from build123d import *

# Parameters (mm, degrees)
F0_R     = 3
F1_DEPTH = 6.4
F4_DEPTH = 3.2
F5_SIZE  = 2


with BuildPart() as f1:
    # F0 (on Top) → F1 (new body)
    with BuildSketch(Plane.XY):
        with BuildLine():
            Line((-69.9830439783, 22.2635182233), (-43.4754125815, 17.5895076134))
            Line((-43.4754125815, 17.5895076134), (-75.4919030254, 33.0095051449))
            ThreePointArc((-75.4919030254, 33.0095051449), (-71.3637669974, 29.3201416884), (-69.8311215084, 24))
            ThreePointArc((-69.8311215084, 24), (-69.8691745275, 23.1284425725), (-69.9830439783, 22.2635182233))
        make_face()
        with BuildLine():
            Line((-90, -10), (-30, -10))
            ThreePointArc((-30, -10), (-37.0710678119, -7.0710678119), (-40, 0))
            Line((-40, 0), (-57, 0))
            ThreePointArc((-57, 0), (-60, -3), (-63, 0))
            Line((-63, 0), (-80, 0))
            ThreePointArc((-80, 0), (-82.9289321881, -7.0710678119), (-90, -10))
        make_face()
        with BuildLine():
            Line((-78.0946397318, 33.8480775301), (-107.6388723221, 39.0575228601))
            ThreePointArc((-107.6388723221, 39.0575228601), (-101.7149096676, 35.6373214269), (-99.3753540988, 29.20944533))
            ThreePointArc((-99.3753540988, 29.20944533), (-99.4134071179, 28.3378879025), (-99.5272765687, 27.4729635533))
            Line((-99.5272765687, 27.4729635533), (-89.6791990386, 25.7364817767))
            ThreePointArc((-89.6791990386, 25.7364817767), (-85.566885872, 32.1915204429), (-78.0946397318, 33.8480775301))
        make_face()
        with BuildLine():
            ThreePointArc((-89.6791990386, 25.7364817767), (-81.5676032851, 14.1519224699), (-69.9830439783, 22.2635182233))
            Line((-69.9830439783, 22.2635182233), (-76.8766982494, 23.479055467))
            ThreePointArc((-76.8766982494, 23.479055467), (-80.3520660414, 21.045576741), (-82.7855447675, 24.520944533))
            Line((-82.7855447675, 24.520944533), (-89.6791990386, 25.7364817767))
        make_face()
        with BuildLine():
            ThreePointArc((-69.8311215084, 24), (-71.3637669974, 29.3201416884), (-75.4919030254, 33.0095051449))
            ThreePointArc((-75.4919030254, 33.0095051449), (-76.7644727965, 33.5181755435), (-78.0946397318, 33.8480775301))
            ThreePointArc((-78.0946397318, 33.8480775301), (-85.566885872, 32.1915204429), (-89.6791990386, 25.7364817767))
            Line((-89.6791990386, 25.7364817767), (-82.7855447675, 24.520944533))
            ThreePointArc((-82.7855447675, 24.520944533), (-79.5696542802, 26.9885840943), (-76.8311215084, 24))
            ThreePointArc((-76.8311215084, 24), (-76.8425374142, 23.7385327718), (-76.8766982494, 23.479055467))
            Line((-76.8766982494, 23.479055467), (-69.9830439783, 22.2635182233))
            ThreePointArc((-69.9830439783, 22.2635182233), (-69.8691745275, 23.1284425725), (-69.8311215084, 24))
        make_face()
        with BuildLine():
            Line((-57, 0), (-40, 0))
            ThreePointArc((-40, 0), (-35.3201416884, 8.467354511), (-25.660781517, 9.0095051449))
            Line((-25.660781517, 9.0095051449), (-43.4754125815, 17.5895076134))
            Line((-43.4754125815, 17.5895076134), (-69.9830439783, 22.2635182233))
            ThreePointArc((-69.9830439783, 22.2635182233), (-81.5676032851, 14.1519224699), (-89.6791990386, 25.7364817767))
            Line((-89.6791990386, 25.7364817767), (-99.5272765687, 27.4729635533))
            ThreePointArc((-99.5272765687, 27.4729635533), (-107.3340404203, 19.4200102868), (-117.7086874321, 23.6817373461))
            Line((-117.7086874321, 23.6817373461), (-102, 0))
            Line((-102, 0), (-98.3333333333, -5.5277079839))
            ThreePointArc((-98.3333333333, -5.5277079839), (-92.8867513459, 9.5742710776), (-80, 0))
            Line((-80, 0), (-63, 0))
            ThreePointArc((-63, 0), (-60, 3), (-57, 0))
        make_face()
        with BuildLine():
            ThreePointArc((-98.3333333333, -5.5277079839), (-94.7287905515, -8.8112734562), (-90, -10))
            ThreePointArc((-90, -10), (-82.9289321881, -7.0710678119), (-80, 0))
            ThreePointArc((-80, 0), (-92.8867513459, 9.5742710776), (-98.3333333333, -5.5277079839))
        make_face()
        with Locations((-90, 0)):
            Circle(F0_R, mode=Mode.SUBTRACT)
        with BuildLine():
            ThreePointArc((-107.6388723221, 39.0575228601), (-117.7409567465, 34.6881944885), (-117.7086874321, 23.6817373461))
            ThreePointArc((-117.7086874321, 23.6817373461), (-107.3340404203, 19.4200102868), (-99.5272765687, 27.4729635533))
            ThreePointArc((-99.5272765687, 27.4729635533), (-99.4134071179, 28.3378879025), (-99.3753540988, 29.20944533))
            ThreePointArc((-99.3753540988, 29.20944533), (-101.7149096676, 35.6373214269), (-107.6388723221, 39.0575228601))
        make_face()
        with BuildLine():
            ThreePointArc((-106.3753540988, 29.20944533), (-106.3867700045, 28.9479781018), (-106.4209308398, 28.688500797))
            ThreePointArc((-106.4209308398, 28.688500797), (-112.3639381931, 29.4709125583), (-106.3753540988, 29.20944533))
        make_face(mode=Mode.SUBTRACT)
        with BuildLine():
            ThreePointArc((-40, 0), (-37.0710678119, -7.0710678119), (-30, -10))
            ThreePointArc((-30, -10), (-22.9289321881, -7.0710678119), (-20, 0))
            Line((-20, 0), (-27, 0))
            ThreePointArc((-27, 0), (-30, -3), (-33, 0))
            Line((-33, 0), (-40, 0))
        make_face()
        with BuildLine():
            Line((-27, 0), (-20, 0))
            ThreePointArc((-20, 0), (-21.532645489, 5.3201416884), (-25.660781517, 9.0095051449))
            ThreePointArc((-25.660781517, 9.0095051449), (-35.3201416884, 8.467354511), (-40, 0))
            Line((-40, 0), (-33, 0))
            ThreePointArc((-33, 0), (-30, 3), (-27, 0))
        make_face()
    extrude(amount=F1_DEPTH)

    # F3 (on offset) → F4 (cut)
    with BuildSketch(Plane.XY.offset(6.4)):
        with BuildLine():
            Line((-121.5190547769, 44.7572868572), (-125.6350207552, 21.4144838341))
            Line((-125.6350207552, 21.4144838341), (-111.1986603593, 18.868963993))
            Line((-111.1986603593, 18.868963993), (-81.6544272584, 13.659518573))
            ThreePointArc((-81.6544272584, 13.659518573), (-86.5803914551, 32.043466615), (-69.3311215084, 24))
            ThreePointArc((-69.3311215084, 24), (-69.3710771859, 23.0848646168), (-69.4906401312, 22.1766939678))
            Line((-69.4906401312, 22.1766939678), (-67.197979989, 35.179015751))
            Line((-67.197979989, 35.179015751), (-121.5190547769, 44.7572868572))
        make_face()
        with BuildLine():
            ThreePointArc((-98.8753540988, 29.20944533), (-102.6260843507, 21.1659785483), (-111.1986603593, 18.868963993))
            ThreePointArc((-111.1986603593, 18.868963993), (-116.1246238469, 37.2529121117), (-98.8753540988, 29.20944533))
        make_face(mode=Mode.SUBTRACT)
        with BuildLine():
            ThreePointArc((-98.8753540988, 29.20944533), (-116.1246238469, 37.2529121117), (-111.1986603593, 18.868963993))
            ThreePointArc((-111.1986603593, 18.868963993), (-102.6260843507, 21.1659785483), (-98.8753540988, 29.20944533))
        make_face()
        with BuildLine():
            ThreePointArc((-69.3311215084, 24), (-86.5803914551, 32.043466615), (-81.6544272584, 13.659518573))
            ThreePointArc((-81.6544272584, 13.659518573), (-73.808568948, 15.3989035201), (-69.4906401312, 22.1766939678))
            ThreePointArc((-69.4906401312, 22.1766939678), (-69.3710771859, 23.0848646168), (-69.3311215084, 24))
        make_face()
        with BuildLine():
            ThreePointArc((-69.4906401312, 22.1766939678), (-73.808568948, 15.3989035201), (-81.6544272584, 13.659518573))
            Line((-81.6544272584, 13.659518573), (-71.3139459673, 11.8362127279))
            Line((-71.3139459673, 11.8362127279), (-69.4906401312, 22.1766939678))
        make_face()
    extrude(amount=-F4_DEPTH, mode=Mode.SUBTRACT)

    # F5
    f5_edges = [f1.edges().sort_by_distance(p)[0] for p in [
        (-50.576342, 21.009505, 0),
        (-46.930289, 19.253468, 6.4),
    ]]
    chamfer(f5_edges, length=F5_SIZE)


with BuildPart() as f6_1:
    # F6: instance of F1
    add(f1.part.mirror(Plane(origin=(-64.9639850302, 5.284700152, 6.4), x_dir=(1, 0, 0), z_dir=(0, 0, 1))))


with BuildPart() as f8_1:
    # F8: instance of F6_1
    add(f6_1.part.mirror(Plane(origin=(-73.367736388, 11.21261041, 12.8), x_dir=(1, 0, 0), z_dir=(0, 0, 1))))


solid = f8_1.part
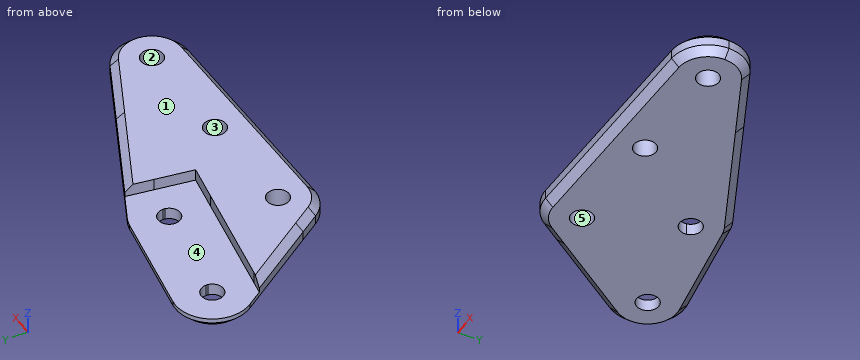
Here's how the part is built. I have some questions about the finished solid (model axes, mm). Face numbers are marked on the shaded views. A direction names the side the tool comes from. Round coordinates to 2 decimals unless told otherwise and drop trailing zeros. Order: outer loops, then holes, each group sorted by start corner. A loop starts at its lowest first (then second) coordinate and runs counter-clockwise, first axis right, second up. Notation, with made-up numbers: (12.5, 4.5) -> (66.5, 4.5) arc R18 cw to (66.5, 31.5) -> close; hole circle Ø8 at (-27.5, 34). An arc over 180 degrees is marked (long way). Use CSV: the item, a comma, the result in double quotes.
1. I need wall thicknesses on line 1 along Y through (x, z) = (-90, 14.5); line 2 along Z through (x, y) = (-74, 24); line 3 along X through (y, z) = (2, 18). Which ranges of each line are inside material? Lowest first, please.
Recorded:
line 1,"y = -9.7 to -3, 3 to 35.64"
line 2,"z = 12.8 to 16"
line 3,"x = -102.37 to -92.24, -87.76 to -62.24, -57.76 to -32.24, -27.76 to -21.02"
2. I'm going to push flat-ended pins straight in: P1, Ø2, axis at x = -105.5, z = 18, coming from the -Y side; P2, Ø2, axis at x = -89, y = 25.5, coming from the +Z side; P3, Ø3.5, axis at x = -60, y = 0, coming from the -Z side; P4, Ø1.5, axis at y = 18.5, z = 17, coming from the +X side. Where does each tip first touch, or does it pass through?
Recorded:
P1,"stops at y = 4.37"
P2,"stops at z = 16"
P3,"passes through"
P4,"stops at x = -43.81"
3. Which directions (+Z, -Z, +X, -X, +Y, -Y) give clear straight access to the entire face, cutting with the end or side of a thin tool? Please do the marked faces 4 and 5.
Recorded:
face 4,"+Z, +Y"
face 5,"+Z, -Z"
4. Thinking about a two-plate mould opening in X: for the marked faces 1, 2 and 3, which applies, pulls with the +X half, pulls with the -X half, needs draft (parallel to the pull), parting line crosses it, or undercut?
Recorded:
face 1,"needs draft"
face 2,"undercut"
face 3,"undercut"
5. I want a section at B-B on x = -49.5. List the corners of the cut face in (y, z) for me, and give its area (3 significant figures).
Recorded:
outline,"(-10, 14.8) -> (-8, 12.8) -> (18.27, 12.8) -> (20.49, 14.8) -> (20.49, 17.2) -> (18.27, 19.2) -> (-8, 19.2) -> (-10, 17.2) -> close"
area,"187 mm2"
6. I want a section at A-A on x = -60. List the corners of the cut face in (y, z) for me, and give its area (3 significant figures).
Recorded:
outline,"(-10, 14.8) -> (-8, 12.8) -> (-3, 12.8) -> (-3, 19.2) -> (-8, 19.2) -> (-10, 17.2) -> close; (3, 12.8) -> (23.33, 12.8) -> (25.55, 14.8) -> (25.55, 17.2) -> (23.33, 19.2) -> (3, 19.2) -> close"
area,"181 mm2"
